```python
from build123d import *

# Parameters (mm, degrees)
F0_R      = 16
F0_R_2    = 10.5
F1_DEPTH  = 20
F2_R      = 12.5
F3_DEPTH  = 15
F4_DEPTH  = 15.001
F5_R      = 14
F6_DEPTH  = 15
F8_W      = 20
F8_H      = 16
F9_DEPTH  = 2
F11_DEPTH = 20
F14_DEPTH = 20
F15_DEPTH = 5.001


with BuildPart() as f1:
    # F0 (on Front) → F1 (new body)
    with BuildSketch(Plane.XZ):
        Circle(F0_R)
        Circle(F0_R_2, mode=Mode.SUBTRACT)
    extrude(amount=F1_DEPTH)

    # F2 (on face) → F3 (join)
    with BuildSketch(Plane.XZ.offset(20)):
        Circle(F2_R)
    extrude(amount=-F3_DEPTH)

    # F4 (cut, through all): a face of the model
    f4_faces = [f1.faces().sort_by_distance(p)[0] for p in [
        (0, -5, 0),
    ]]
    extrude(f4_faces, amount=-F4_DEPTH, mode=Mode.SUBTRACT)

    # F5 (on face) → F6 (cut)
    with BuildSketch(Plane(origin=(0, 0, 0), x_dir=(-1, 0, 0), z_dir=(0, 1, 0))):
        Circle(F5_R)
    extrude(amount=-F6_DEPTH, mode=Mode.SUBTRACT)

    # F8 (on offset) → F9 (join)
    with BuildSketch(Plane.YZ.offset(15)):
        with Locations((-10, -8)):
            Rectangle(F8_W, F8_H)
        with Locations((-10, 8)):
            Rectangle(F8_W, F8_H)
    extrude(amount=F9_DEPTH)

    # F10 (on face) → F11 (join)
    with BuildSketch(Plane.XZ.offset(20)):
        with BuildLine():
            Line((15, 16), (0, 16))
            ThreePointArc((0, 16), (9.1355287257, 13.1355287257), (15, 5.5677643628))
            Line((15, 5.5677643628), (15, 16))
        make_face()
    extrude(amount=-F11_DEPTH)

    # F13 (on face) → F14 (join)
    with BuildSketch(Plane.XZ.offset(20)):
        with BuildLine():
            Line((0, -16), (15, -16))
            Line((15, -16), (15, -5.5677643628))
            ThreePointArc((15, -5.5677643628), (9.1355287257, -13.1355287257), (0, -16))
        make_face()
    extrude(amount=-F14_DEPTH)

    # F15 (cut, through all): a face of the model
    f15_faces = [f1.faces().sort_by_distance(p)[0] for p in [
        (13.6040202025, -15, 0),
    ]]
    extrude(f15_faces, amount=-F15_DEPTH, mode=Mode.SUBTRACT)


solid = f1.part
```
Geometry check sheet. Reference: the model listing, model coordinates, mm. Give positions to 0.01 mm unless a question says otherwise; leave off trailing zeros. Write each loop counter-clockwise with the first axis right and the second up, starting at its lowest first coordinate (ties: lowest second). Pieces come first, ordered by that corner, then holes. Notation, with made-up numbers: (33, 31) - (90, 31) arc R10 cw to (90, 40) - close; hole circle Ø6 at (-23, 53.25). An arc over 180 degrees is marked (long way). Use a Markdown table: item, result.
Q1. Section check B-B, the plane x = -7. Enter the section's corners in (y, z).
Computed:
| item | result |
|---|---|
| outline | (-20, -14.39) - (0, -14.39) - (0, -12.12) - (-20, -12.12) - close; (-20, 12.12) - (0, 12.12) - (0, 14.39) - (-20, 14.39) - close |
Q2. Section check C-C, the plane y = -8. Enter the section's corners in (x, z), then the cut area to 3 significant figures.
Computed:
| item | result |
|---|---|
| outline | (0, -16) - (17, -16) - (17, 16) - (0, 16) arc R16 ccw to start; hole circle Ø28 at (0, 0) |
| area | 330 mm² |
Q3. Draft check along Z on faces 1 (the face through (14, -20, -5)), 2 (the face through (-16, -10, 0)), 3 (the face through (-12.932, -9.86, -5.362)). Enter one of: pulls with the +Z half, pulls with the -Z half, needs draft (parallel to the pull), parting line crosses it, or undercut.
Computed:
| item | result |
|---|---|
| face 1 | needs draft |
| face 2 | parting line crosses it |
| face 3 | undercut |
Q4. Thickness scan on L1, parallel to X at y = -13.25, z = -0.5; L2, parallel to Z at x = -2.5, y = -9.25; L3, parallel to Z at x = -11, y = -1.25. Record the ranges inside material, lowest first. Write a range as [from, to].
Computed:
| item | result |
|---|---|
| L1 | x = [-15.99, -13.99], [13.99, 17] |
| L2 | z = [-15.8, -13.77], [13.77, 15.8] |
| L3 | z = [-11.62, -8.66], [8.66, 11.62] |
Q5. Go/stop test with flat-tipped pins: P1, Ø6, axis at x = 8, z = -9, coming from the -Y side; P2, Ø3, axis at y = -15.5, z = 4, coming from the -X side; P3, Ø1.5, axis at y = -16.5, z = -5, coming from the -X side; P4, Ø2, axis at y = -8, z = 10, coming from the -X side. Record where each tip stops, or that it passes through.
Computed:
| item | result |
|---|---|
| P1 | stops at y = -20 |
| P2 | stops at x = -15.8 |
| P3 | stops at x = -15.43 |
| P4 | stops at x = -13.23 |
Q6. Section check A-A, the plane z = 0. Enter the section's corners in (x, y).
Computed:
| item | result |
|---|---|
| outline | (-16, -20) - (-14, -20) - (-14, 0) - (-16, 0) - close; (14, -20) - (17, -20) - (17, 0) - (14, 0) - close |
